Work out the finished part from the listing and answer in its coordinate system (mm). A direction names the side the tool comes from. Round coordinates to 2 decimals unless told otherwise and drop trailing zeros. Order: outer loops, then holes, each group sorted by start corner. A loop starts at its lowest first (then second) coordinate and runs counter-clockwise, first axis right, second up. Notation, with made-up numbers: M 42.25,88.25 L 57.25,88.25 A9 cw 57.25,105.25 Z; hole C 63,57 d1. An arc over 180 degrees is marked long. Return JSON: item names as keys, results as strings.
from build123d import *

# Parameters (mm, degrees)
SKETCH1_R           = 2.286
MAIN_BODY_DEPTH     = 1.5875
SKETCH3_R           = 2.286
BOSS_EXTRUDE1_DEPTH = 6.35
CUT_EXTRUDE2_REACH  = 3.587
SKETCH2_W           = 6.35
SKETCH2_H           = 1.5875
SKETCH5_W           = 6.35
SKETCH5_H           = 1.5875
BOSS_EXTRUDE3_DEPTH = 1.5875


with BuildPart() as part:
    # Sketch1 → Main Body (new body)
    with BuildSketch(Plane(origin=(0, 0, 0), x_dir=(1, 0, 0), z_dir=(0, 1, 0))):
        Polygon((-25.4, 86.995), (-63.43142, 86.995), (-63.43142, 60.96), (-78.74, 60.96), (-78.74, 25.4), (-71.12, 25.4), (-71.12, -25.4), (-78.74, -25.4), (-78.74, -60.96), (-63.43142, -60.96), (-63.43142, -86.995), (-25.4, -86.995), (-25.4, -79.375), (25.4, -79.375), (25.4, -86.995), (63.43142, -86.995), (63.43142, -60.96), (78.74, -60.96), (78.74, -25.4), (71.12, -25.4), (71.12, 25.4), (78.74, 25.4), (78.74, 60.96), (63.43142, 60.96), (63.43142, 86.995), (25.4, 86.995), (25.4, 79.375), (-25.4, 79.375), align=None)
        with Locations((-57.15, 76.2)):
            Circle(SKETCH1_R, mode=Mode.SUBTRACT)
        with Locations((57.15, 76.2)):
            Circle(SKETCH1_R, mode=Mode.SUBTRACT)
        with Locations((57.15, -76.2)):
            Circle(SKETCH1_R, mode=Mode.SUBTRACT)
        with Locations((-57.15, -76.2)):
            Circle(SKETCH1_R, mode=Mode.SUBTRACT)
    extrude(amount=MAIN_BODY_DEPTH)

    # Sketch3 → Boss-Extrude1 (add)
    with BuildSketch(Plane(origin=(0, 1.5875, 0), x_dir=(1, 0, 0), z_dir=(0, 1, 0))):
        with BuildLine():
            Line((62.175136, -72.431148), (7.851775, 0))
            Line((7.851775, 0), (62.175136, 72.431148))
            ThreePointArc((62.175136, 72.431148), (60.918852, 81.225136), (52.124864, 79.968852))
            Line((52.124864, 79.968852), (0, 10.469033333))
            Line((0, 10.469033333), (-52.124864, 79.968852))
            ThreePointArc((-52.124864, 79.968852), (-60.918852, 81.225136), (-62.175136, 72.431148))
            Line((-62.175136, 72.431148), (-7.851775, 0))
            Line((-7.851775, 0), (-62.175136, -72.431148))
            ThreePointArc((-62.175136, -72.431148), (-60.918852, -81.225136), (-52.124864, -79.968852))
            Line((-52.124864, -79.968852), (0, -10.469033333))
            Line((0, -10.469033333), (52.124864, -79.968852))
            ThreePointArc((52.124864, -79.968852), (60.918852, -81.225136), (62.175136, -72.431148))
        make_face()
        with Locations((57.15, 76.2)):
            Circle(SKETCH3_R, mode=Mode.SUBTRACT)
        with Locations((57.15, -76.2)):
            Circle(SKETCH3_R, mode=Mode.SUBTRACT)
        with Locations((-57.15, -76.2)):
            Circle(SKETCH3_R, mode=Mode.SUBTRACT)
        with Locations((-57.15, 76.2)):
            Circle(SKETCH3_R, mode=Mode.SUBTRACT)
    extrude(amount=BOSS_EXTRUDE1_DEPTH)

    # Sketch2 → Cut-Extrude2 (cut, up to next)
    with BuildSketch(Plane(origin=(0, 1.5875, 0), x_dir=(1, 0, 0), z_dir=(0, 1, 0)), mode=Mode.PRIVATE) as cut_extrude2_sk1:
        with Locations((0.508, -67.78625)):
            Rectangle(SKETCH2_W, SKETCH2_H)
    cut_extrude2_tool1 = extrude(cut_extrude2_sk1.sketch, amount=-CUT_EXTRUDE2_REACH, mode=Mode.PRIVATE) & part.part
    add(cut_extrude2_tool1.solids().sort_by_distance((0.508, 1.5875, 67.78625))[0], mode=Mode.SUBTRACT)
    # Sketch2 → Cut-Extrude2 (cut, up to next)
    with BuildSketch(Plane(origin=(0, 1.5875, 0), x_dir=(1, 0, 0), z_dir=(0, 1, 0)), mode=Mode.PRIVATE) as cut_extrude2_sk2:
        with Locations((0.508, -73.18375)):
            Rectangle(SKETCH2_W, SKETCH2_H)
    cut_extrude2_tool2 = extrude(cut_extrude2_sk2.sketch, amount=-CUT_EXTRUDE2_REACH, mode=Mode.PRIVATE) & part.part
    add(cut_extrude2_tool2.solids().sort_by_distance((0.508, 1.5875, 73.18375))[0], mode=Mode.SUBTRACT)
    # Sketch2 → Cut-Extrude2 (cut, up to next)
    with BuildSketch(Plane(origin=(0, 1.5875, 0), x_dir=(1, 0, 0), z_dir=(0, 1, 0)), mode=Mode.PRIVATE) as cut_extrude2_sk3:
        with Locations((27.305, -67.78625)):
            Rectangle(SKETCH2_W, SKETCH2_H)
    cut_extrude2_tool3 = extrude(cut_extrude2_sk3.sketch, amount=-CUT_EXTRUDE2_REACH, mode=Mode.PRIVATE) & part.part
    add(cut_extrude2_tool3.solids().sort_by_distance((27.305, 1.5875, 67.78625))[0], mode=Mode.SUBTRACT)
    # Sketch2 → Cut-Extrude2 (cut, up to next)
    with BuildSketch(Plane(origin=(0, 1.5875, 0), x_dir=(1, 0, 0), z_dir=(0, 1, 0)), mode=Mode.PRIVATE) as cut_extrude2_sk4:
        with Locations((27.305, -73.18375)):
            Rectangle(SKETCH2_W, SKETCH2_H)
    cut_extrude2_tool4 = extrude(cut_extrude2_sk4.sketch, amount=-CUT_EXTRUDE2_REACH, mode=Mode.PRIVATE) & part.part
    add(cut_extrude2_tool4.solids().sort_by_distance((27.305, 1.5875, 73.18375))[0], mode=Mode.SUBTRACT)
    # Sketch2 → Cut-Extrude2 (cut, up to next)
    with BuildSketch(Plane(origin=(0, 1.5875, 0), x_dir=(1, 0, 0), z_dir=(0, 1, 0)), mode=Mode.PRIVATE) as cut_extrude2_sk5:
        with Locations((0.508, 67.78625)):
            Rectangle(SKETCH2_W, SKETCH2_H)
    cut_extrude2_tool5 = extrude(cut_extrude2_sk5.sketch, amount=-CUT_EXTRUDE2_REACH, mode=Mode.PRIVATE) & part.part
    add(cut_extrude2_tool5.solids().sort_by_distance((0.508, 1.5875, -67.78625))[0], mode=Mode.SUBTRACT)
    # Sketch2 → Cut-Extrude2 (cut, up to next)
    with BuildSketch(Plane(origin=(0, 1.5875, 0), x_dir=(1, 0, 0), z_dir=(0, 1, 0)), mode=Mode.PRIVATE) as cut_extrude2_sk6:
        with Locations((0.508, 73.18375)):
            Rectangle(SKETCH2_W, SKETCH2_H)
    cut_extrude2_tool6 = extrude(cut_extrude2_sk6.sketch, amount=-CUT_EXTRUDE2_REACH, mode=Mode.PRIVATE) & part.part
    add(cut_extrude2_tool6.solids().sort_by_distance((0.508, 1.5875, -73.18375))[0], mode=Mode.SUBTRACT)
    # Sketch2 → Cut-Extrude2 (cut, up to next)
    with BuildSketch(Plane(origin=(0, 1.5875, 0), x_dir=(1, 0, 0), z_dir=(0, 1, 0)), mode=Mode.PRIVATE) as cut_extrude2_sk7:
        with Locations((27.305, 73.18375)):
            Rectangle(SKETCH2_W, SKETCH2_H)
    cut_extrude2_tool7 = extrude(cut_extrude2_sk7.sketch, amount=-CUT_EXTRUDE2_REACH, mode=Mode.PRIVATE) & part.part
    add(cut_extrude2_tool7.solids().sort_by_distance((27.305, 1.5875, -73.18375))[0], mode=Mode.SUBTRACT)
    # Sketch2 → Cut-Extrude2 (cut, up to next)
    with BuildSketch(Plane(origin=(0, 1.5875, 0), x_dir=(1, 0, 0), z_dir=(0, 1, 0)), mode=Mode.PRIVATE) as cut_extrude2_sk8:
        with Locations((27.305, 67.78625)):
            Rectangle(SKETCH2_W, SKETCH2_H)
    cut_extrude2_tool8 = extrude(cut_extrude2_sk8.sketch, amount=-CUT_EXTRUDE2_REACH, mode=Mode.PRIVATE) & part.part
    add(cut_extrude2_tool8.solids().sort_by_distance((27.305, 1.5875, -67.78625))[0], mode=Mode.SUBTRACT)

    # Sketch5 → Boss-Extrude3 (add)
    with BuildSketch(Plane(origin=(0, 1.5875, 0), x_dir=(1, 0, 0), z_dir=(0, 1, 0))):
        Polygon((-4.2545, -70.8025), (-4.2545, -70.1675), (-4.2545, -65.405), (5.2705, -65.405), (5.2705, -70.1675), (5.2705, -70.8025), (5.2705, -75.565), (-4.2545, -75.565), align=None)
        with Locations((0.508, -67.78625)):
            Rectangle(SKETCH5_W, SKETCH5_H, mode=Mode.SUBTRACT)
        with Locations((0.508, -73.18375)):
            Rectangle(SKETCH5_W, SKETCH5_H, mode=Mode.SUBTRACT)
        Polygon((22.5425, -70.8025), (22.5425, -70.1675), (22.5425, -65.405), (32.0675, -65.405), (32.0675, -70.1675), (32.0675, -70.8025), (32.0675, -75.565), (22.5425, -75.565), align=None)
        with Locations((27.305, -67.78625)):
            Rectangle(SKETCH5_W, SKETCH5_H, mode=Mode.SUBTRACT)
        with Locations((27.305, -73.18375)):
            Rectangle(SKETCH5_W, SKETCH5_H, mode=Mode.SUBTRACT)
        Polygon((-4.2545, 65.405), (5.2705, 65.405), (5.2705, 70.1675), (5.2705, 70.8025), (5.2705, 75.565), (-4.2545, 75.565), (-4.2545, 70.8025), (-4.2545, 70.1675), align=None)
        with Locations((0.508, 73.18375)):
            Rectangle(SKETCH5_W, SKETCH5_H, mode=Mode.SUBTRACT)
        with Locations((0.508, 67.78625)):
            Rectangle(SKETCH5_W, SKETCH5_H, mode=Mode.SUBTRACT)
        Polygon((22.5425, 65.405), (32.0675, 65.405), (32.0675, 70.1675), (32.0675, 70.8025), (32.0675, 75.565), (22.5425, 75.565), (22.5425, 70.8025), (22.5425, 70.1675), align=None)
        with Locations((27.305, 73.18375)):
            Rectangle(SKETCH5_W, SKETCH5_H, mode=Mode.SUBTRACT)
        with Locations((27.305, 67.78625)):
            Rectangle(SKETCH5_W, SKETCH5_H, mode=Mode.SUBTRACT)
    extrude(amount=BOSS_EXTRUDE3_DEPTH)


solid = part.part
Item 1: Find section C-C (x = -34). Determine the outline of the cut face in (y, z) (1 decimal), plus the area to 3 significant figures.
Output:
{"outline": "M 0,-87 L 1.6,-87 L 1.6,-55.8 L 7.9,-55.8 L 7.9,-34.9 L 1.6,-34.9 L 1.6,34.9 L 7.9,34.9 L 7.9,55.8 L 1.6,55.8 L 1.6,87 L 0,87 Z", "area": "542 mm^2"}
Item 2: Consider line 1 along X through (y, z) = (3.75, -76.2); line 2 along Y through (x, z) = (32.5, -78); line 3 along Z through (x, y) = (57.15, 5.5). Determine where each line is inside the solid, lowest interval first. Write a range as [from, to].
Output:
{"line 1": "x = [-63.43, -59.44], [-54.86, -49.3], [49.3, 54.86], [59.44, 63.43]", "line 2": "y = [0, 1.59]", "line 3": "z = [-82.48, -78.49], [-73.91, -65.73], [65.73, 73.91], [78.49, 82.48]"}
Item 3: Which of the six approach directions +Z, -Z, +X, -X, +Y, -Y give full straight-line access (tool end or side, diameter ignored) to faces 1 (the flat face through (27, 3.175, -71)), 2 (the cylindrical face through (-60.807, 4.718, -81.307)), 3 (the flat face through (51, 1.588, -1))?
Output:
{"face 1": "-Z, +Y", "face 2": "+Y", "face 3": "+X, +Y"}
Item 4: Find section B-B (x = 57.15). Determine the outline of the cut face in (y, z) (1 decimal), plus the area to 3 significant figures.
Output:
{"outline": "M 0,-87 L 1.6,-87 L 1.6,-82.5 L 7.9,-82.5 L 7.9,-78.5 L 0,-78.5 Z; M 0,-73.9 L 7.9,-73.9 L 7.9,-65.7 L 1.6,-65.7 L 1.6,65.7 L 7.9,65.7 L 7.9,73.9 L 0,73.9 Z; M 0,78.5 L 7.9,78.5 L 7.9,82.5 L 1.6,82.5 L 1.6,87 L 0,87 Z", "area": "416 mm^2"}
Item 5: Each of these flat-tipped pins is pushed along its axis until it touches: pin 1 (0.8 mm diameter, centred on y = 3, z = 72, fed in from +X); pin 2 (1.6 mm diameter, centred on x = 0.5, y = 2, fed in from -Z) (3 decimals); pin 3 (1.7 mm diameter, centred on y = 2.5, z = 73.5, fed in from +X). Where does it stop, or does it pass through?
Output:
{"pin 1": "stops at x = 62.15", "pin 2": "stops at z = -79.375", "pin 3": "stops at x = 63.15"}
Item 6: Find section D-D (z = 32.5). Determine the outline of the cut face in (x, y).
Output:
{"outline": "M -78.74,0 L 78.74,0 L 78.74,1.59 L 32.23,1.59 L 32.23,7.94 L 16.52,7.94 L 16.52,1.59 L -16.52,1.59 L -16.52,7.94 L -32.23,7.94 L -32.23,1.59 L -78.74,1.59 Z"}
Item 7: Find section A-A (y = 5). Determine the outline of the cut face in (x, z).
Output:
{"outline": "M -62.18,-72.43 A6.28 ccw -52.12,-79.97 L 0,-10.47 L 52.12,-79.97 A6.28 ccw 62.18,-72.43 L 7.85,0 L 62.18,72.43 A6.28 ccw 52.12,79.97 L 0,10.47 L -52.12,79.97 A6.28 ccw -62.18,72.43 L -7.85,0 Z; hole C -57.15,-76.2 d4.57; hole C -57.15,76.2 d4.57; hole C 57.15,-76.2 d4.57; hole C 57.15,76.2 d4.57"}
